CAD build for the part. Positions are in the model's coordinates, mm. A direction names the side the tool comes from. Round coordinates to 2 decimals unless told otherwise and drop trailing zeros. Loops run counter-clockwise (first coordinate to the right, second up) from the corner with the lowest first, then second, coordinate; pieces in that order, holes last. Notation, with made-up numbers: (60.5, -7) - (92.5, -7) arc R21 cw to (92.5, 9) - close; hole circle Ø10 at (10, 2). An arc over 180 degrees is marked (long way). Use one line per item in the form item = value.
Solid Edge part; units mm, degrees
sketch "Sketch1" plane through (0, 0, 0) normal (0, -1, 0) x (1, 0, 0)
  line L0 (66.5, 100) -> (-66.5, 100)
  line L1 (-66.5, 100) -> (-66.5, -100)
  line L2 (-66.5, -100) -> (66.5, -100)
  line L3 (66.5, -100) -> (66.5, 100)
  line L4 (81.5, 115) -> (-81.5, 115)
  line L5 (-81.5, 115) -> (-81.5, -115)
  line L6 (-81.5, -115) -> (81.5, -115)
  line L7 (81.5, -115) -> (81.5, 115)
extrude "Protrusion1" add sketch "Sketch1" along normal blind 15
chamfer "Fase_1" distance 15 angle 45 4 edges at (-81.5, -15, 0) (0, -15, 115) (81.5, -15, 0) (0, -15, -115)
1) Tool access for faces 4 (the flat face through (-71, 0, 2)), 5 (the flat face through (-66.5, -7, 1)): list every direction of +Z, -Z, +X, -X, +Y, -Y with a clear straight run to the whole face (end or side of a thin tool).
Report:
face_4 = +Z, -Z, +X, -X, +Y
face_5 = +Y, -Y
2) Slice it at C-C (y = -8.5). Write the cut outline in (x, z), plus the area to 3 significant figures.
Report:
outline = (-73, -106.5) - (73, -106.5) - (73, 106.5) - (-73, 106.5) - close; hole (-66.5, -100) - (66.5, -100) - (66.5, 100) - (-66.5, 100) - close
area = 4,500 mm^2
3) Drill centre lines: probe 1 along Z at (x, y) = (-34, -9.25); probe 2 along X at (y, z) = (-13.75, -84.5); probe 3 along Z at (x, y) = (61, -4.75). Where is each one in solid material? Low to high.
Report:
probe_1 = -105.75 to -100, 100 to 105.75
probe_2 = -67.75 to -66.5, 66.5 to 67.75
probe_3 = -110.25 to -100, 100 to 110.25
4) Two-plate mould, pull along X, no slides. Class faces 1 (the flat face through (66.5, -7, -1)), 2 (the flat face through (1, -8, -107)), 3 (the flat face through (73.9, -7.6, 1.6)): +X half, -X half, draft (parallel to the pull), parting line (faces both ways), or undercut.
Report:
face_1 = undercut
face_2 = draft
face_3 = +X half
5) Flat gauge pins, fed straight in: pin 1 (8 mm diameter, centred on x = 11.5, y = -9, fed in from +Z); pin 2 (3 mm diameter, centred on x = -8.5, y = -12.5, fed in from +Z); pin 3 (4 mm diameter, centred on y = -9.5, z = 38, fed in from +X). Where does each tip first touch, or does it go through?
Report:
pin_1 = 110
pin_2 = 104
pin_3 = 74
